Answer from the drawing. Dimensions are ordinates in mm from the lowest x, y and z of the part. A direction names the side the tool comes from. Give positions to 0.01 mm unless a question says otherwise; leave off trailing zeros. Order: outer loops, then holes, each group sorted by start corner. A loop starts at its lowest first (then second) coordinate and runs counter-clockwise, first axis right, second up. Notation, with made-up numbers: (58, 51) - (92, 51) arc R10 ccw to (92, 61) - close; hole circle Ø4 at (-34.75, 61). An arc over 180 degrees is marked (long way). Write each question's results on one line, items separated by ' | '.
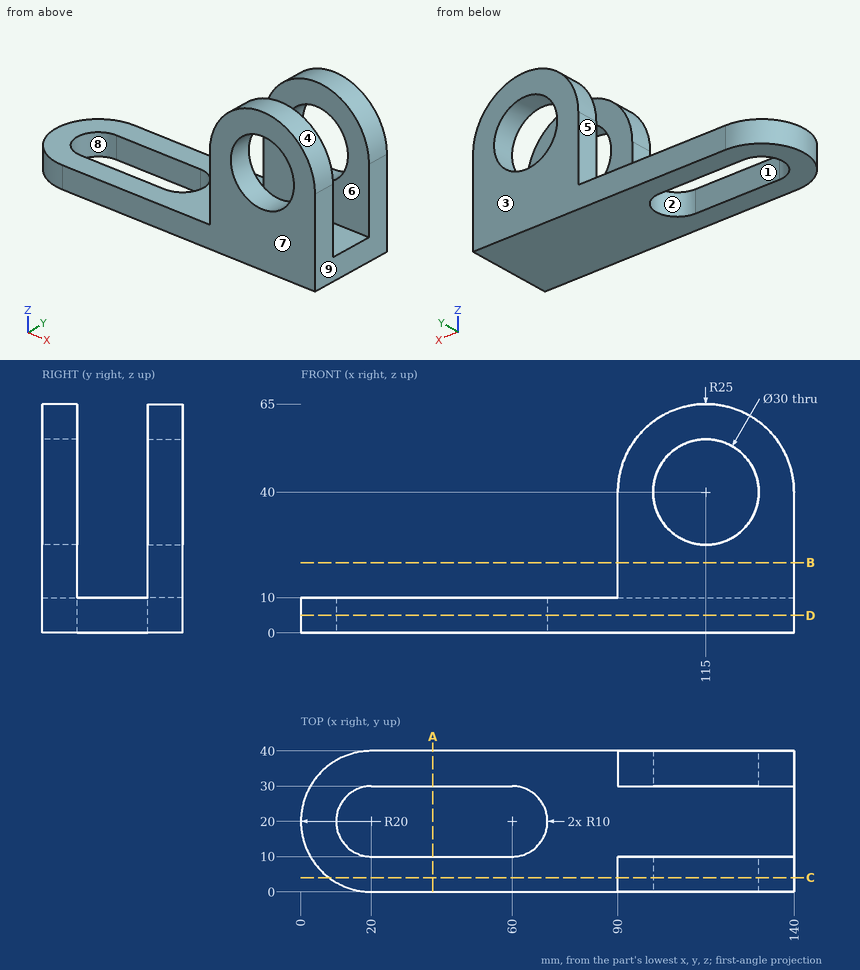
1. A cutting plane is placed at B-B, the plane z = 20. Write down the section's boundary in (x, y), then the cut area to 3 significant figures.
Answer list:
outline: (90, 0) - (140, 0) - (140, 10) - (90, 10) - close; (90, 30) - (140, 30) - (140, 40) - (90, 40) - close | area: 1,000 mm^2
2. A cutting plane is placed at C-C, the plane y = 4. Write down the section's boundary in (x, z).
Answer list:
outline: (8, 0) - (140, 0) - (140, 40) arc R25 ccw to (90, 40) - (90, 10) - (8, 10) - close; hole circle Ø30 at (115, 40)
3. Straight lines are drawn through the part: line 1 (Z direction, x = 115, y = 5); line 2 (X direction, y = 2.5, z = 40); line 3 (Y direction, x = 99.5, z = 16.5). For each, find the intervals that lie inside material, in ascending order. Write a range as [from, to].
Answer list:
line 1: [0, 25], [55, 65] | line 2: [90, 100], [130, 140] | line 3: [0, 10], [30, 40]
4. A tool of negligible diameter and unlimited length cuts with its end or side. For the marked faces 5, 6, 7, 8 and 9, from which of +Z, -Z, +X, -X, +Y, -Y can it reach the whole face along a straight path? Write none if from no direction.
Answer list:
face 5: +Z, -X, +Y, -Y | face 6: +Z, +X, -X | face 7: +Z, -Z, +X, -X, -Y | face 8: +Z, -Z | face 9: +Z, -Z, +X, +Y, -Y
5. Determine the mould class of the marked faces 1, 2, 3 and 4 for opening direction X: +X half, -X half, draft (parallel to the pull), parting line (faces both ways), or undercut.
Answer list:
face 1: undercut | face 2: undercut | face 3: draft | face 4: parting line
6. A cutting plane is placed at D-D, the plane z = 5. Write down the section's boundary in (x, y).
Answer list:
outline: (20, 0) - (140, 0) - (140, 40) - (20, 40) arc R20 ccw to start; hole (20, 10) - (60, 10) arc R10 ccw to (60, 30) - (20, 30) arc R10 ccw to start
7. A cutting plane is placed at A-A, the plane x = 37.5. Write down the section's boundary in (y, z), then the cut area to 3 significant figures.
Answer list:
outline: (0, 0) - (10, 0) - (10, 10) - (0, 10) - close; (30, 0) - (40, 0) - (40, 10) - (30, 10) - close | area: 200 mm^2
8. Given P1, Ø11, axis at y = 3.5, z = 18.5, coming from the -X side; P2, Ø4, axis at x = 18, y = 27, coming from the +Z side; P3, Ø15, axis at x = 107.5, z = 34.5, coming from the -Y side; P4, Ø12, axis at x = 102, y = 20, coming from the +Z side, each flat-ended and moving along its own axis, determine where each tip first touches the part or whether it passes through.
Answer list:
P1: x = 90 | P2: through | P3: y = 0 | P4: z = 10
